```python
from build123d import *

# Parameters (mm, degrees)
F0_R            = 38.1
F1_DEPTH        = 6.35
F2_R            = 3.175
F3_DEPTH        = 6.351
F3_COPIES_COUNT = 8
F5_DEPTH        = 25.4


# Not quite as in the source:
# - a pattern or mirror of a feature is missing from the dataset's text; its kind, count and spacing are read off the source's solid


with BuildPart() as f1:
    # F0 (on Front) → F1 (new body)
    with BuildSketch(Plane.XZ):
        Circle(F0_R)
    extrude(amount=F1_DEPTH)

    # F2 (on face) → F3 (cut, through all)
    with BuildSketch(Plane.XZ.offset(6.35)):
        with Locations((0, 31.6533222795)):
            Circle(F2_R)
    f3 = extrude(amount=-F3_DEPTH, mode=Mode.SUBTRACT)

    # F3_copies: F3 ×8 about axis
    f3_copies_axis = Axis((0, 0, 0), (0, 1, 0))
    for i in range(1, F3_COPIES_COUNT):
        add(f3.rotate(f3_copies_axis, i * 360 / F3_COPIES_COUNT), mode=Mode.SUBTRACT)

    # F4 (on Front) → F5 (intersect)
    with BuildSketch(Plane.XZ):
        with BuildLine():
            Line((3.1097339764, 36.7998792025), (-3.5963490721, 36.7998792025))
            Line((-3.5963490721, 36.7998792025), (-7.5950432294, 25.4702454258))
            ThreePointArc((-7.5950432294, 25.4702454258), (-10.1728112394, 24.5546735917), (-12.6428176097, 23.378991565))
            Line((-12.6428176097, 23.378991565), (-23.8225301486, 28.2203581134))
            Line((-23.8225301486, 28.2203581134), (-28.5644469474, 23.4784413146))
            Line((-28.5644469474, 23.4784413146), (-23.38068983, 12.6396766882))
            ThreePointArc((-23.38068983, 12.6396766882), (-24.5560400177, 10.1695123954), (-25.4712655381, 7.5916214078))
            Line((-25.4712655381, 7.5916214078), (-36.7998792025, 3.1097339764))
            Line((-36.7998792025, 3.1097339764), (-36.7998792025, -3.5963490721))
            Line((-36.7998792025, -3.5963490721), (-25.4702454258, -7.5950432294))
            ThreePointArc((-25.4702454258, -7.5950432294), (-24.5546735917, -10.1728112394), (-23.378991565, -12.6428176097))
            Line((-23.378991565, -12.6428176097), (-28.2203581134, -23.8225301486))
            Line((-28.2203581134, -23.8225301486), (-23.4784413146, -28.5644469474))
            Line((-23.4784413146, -28.5644469474), (-12.6396766882, -23.38068983))
            ThreePointArc((-12.6396766882, -23.38068983), (-10.1695123954, -24.5560400177), (-7.5916214078, -25.4712655381))
            Line((-7.5916214078, -25.4712655381), (-3.1097339764, -36.7998792025))
            Line((-3.1097339764, -36.7998792025), (3.5963490721, -36.7998792025))
            Line((3.5963490721, -36.7998792025), (7.5950432294, -25.4702454258))
            ThreePointArc((7.5950432294, -25.4702454258), (10.1728112394, -24.5546735917), (12.6428176097, -23.378991565))
            Line((12.6428176097, -23.378991565), (23.8225301486, -28.2203581134))
            Line((23.8225301486, -28.2203581134), (28.5644469474, -23.4784413146))
            Line((28.5644469474, -23.4784413146), (23.38068983, -12.6396766882))
            ThreePointArc((23.38068983, -12.6396766882), (24.5560400177, -10.1695123954), (25.4712655381, -7.5916214078))
            Line((25.4712655381, -7.5916214078), (36.7998792025, -3.1097339764))
            Line((36.7998792025, -3.1097339764), (36.7998792025, 3.5963490721))
            Line((36.7998792025, 3.5963490721), (25.4702454258, 7.5950432294))
            ThreePointArc((25.4702454258, 7.5950432294), (24.5546735917, 10.1728112394), (23.378991565, 12.6428176097))
            Line((23.378991565, 12.6428176097), (28.2203581134, 23.8225301486))
            Line((28.2203581134, 23.8225301486), (23.4784413146, 28.5644469474))
            Line((23.4784413146, 28.5644469474), (12.6396766882, 23.38068983))
            ThreePointArc((12.6396766882, 23.38068983), (10.1695123954, 24.5560400177), (7.5916214078, 25.4712655381))
            Line((7.5916214078, 25.4712655381), (3.1097339764, 36.7998792025))
        make_face()
    extrude(amount=F5_DEPTH, mode=Mode.INTERSECT)


solid = f1.part
```
Check sheet for the modelled part. Datum: model origin and axes. Units: mm. A direction names the side the tool comes from. Round coordinates to 2 decimals unless told otherwise and drop trailing zeros. Write each loop counter-clockwise with the first axis right and the second up, starting at its lowest first coordinate (ties: lowest second). Pieces come first, ordered by that corner, then holes. Notation, with made-up numbers: (86.5, 29.25) -> (110.5, 29.25) arc R21 cw to (110.5, 62.25) -> close; hole circle Ø3 at (-26.5, -27.5). An arc over 180 degrees is marked (long way). One line per question, with ' | ' between items. Start each with the question number.
1. Sectioned sample at C-C, the plane z = 30.5. Record the cut outline in (x, y), then the cut area to 3 significant figures.
2. Release check for a two-part mould opening along X. For faces 1 (the face through (31.06, -3.13, -5.38)), 2 (the face through (-18.154, -3.131, 25.766)), 3 (the face through (0, -3, 36.8)) record: +X half, -X half, draft (parallel to the pull), parting line (faces both ways), or undercut.
3. Set-up check for faces 4 (the face through (25.766, -3.131, 18.154)), 5 (the face through (-5.57, -3.13, 31.21)), 6 (the face through (-18.135, -3.131, -26.009)): record each of +Z, -Z, +X, -X, +Y, -Y from which the full face is reachable in a straight line by a thin tool's end or side.
4. Scan lines: line 1 along X through (y, z) = (-3.5, 0); line 2 along X through (y, z) = (-1.5, 2.5). Record each from-to range of solid material in increasing order. Write a range as from..to.
5. Sectioned sample at A-A, the plane z = 0. Record the cut outline in (x, y), then the cut area to 3 significant figures.
6. Sectioned sample at B-B, the plane x = 0. Record the cut outline in (y, z), then the cut area to 3 significant figures.
7. Sectioned sample at D-D, the plane y = -2.25. Count the separate pieces of the cut face and the enclosed holes in it, then the cut area to 3 significant figures.
Taken from the geometry:
1) outline: (-5.82, -6.35) -> (-2.96, -6.35) -> (-2.96, 0) -> (-5.82, 0) -> close; (2.96, -6.35) -> (5.6, -6.35) -> (5.6, 0) -> (2.96, 0) -> close | area: 35.0 mm^2
2) face 1: +X half | face 2: undercut | face 3: draft
3) face 4: +X, +Y, -Y | face 5: +Z, +Y, -Y | face 6: -Z, +Y, -Y
4) line 1: x = -36.8..-34.83, -28.48..28.48, 34.83..36.8 | line 2: x = -36.8..-33.61, -29.7..29.7, 33.61..36.8
5) outline: (-36.8, -6.35) -> (-34.83, -6.35) -> (-34.83, 0) -> (-36.8, 0) -> close; (-28.48, -6.35) -> (28.48, -6.35) -> (28.48, 0) -> (-28.48, 0) -> close; (34.83, -6.35) -> (36.8, -6.35) -> (36.8, 0) -> (34.83, 0) -> close | area: 387 mm^2
6) outline: (-6.35, -36.8) -> (0, -36.8) -> (0, -34.83) -> (-6.35, -34.83) -> close; (-6.35, -28.48) -> (0, -28.48) -> (0, 28.48) -> (-6.35, 28.48) -> close; (-6.35, 34.83) -> (0, 34.83) -> (0, 36.8) -> (-6.35, 36.8) -> close | area: 387 mm^2
7) separate pieces: 1 | enclosed holes: 8 | area: 2,870 mm^2
